Can you work these out from the model? Positions are in its coordinate system, mm. A direction names the side the tool comes from. Give positions to 0.01 mm unless a question says otherwise; leave off trailing zeros. Order: outer loops, then holes, each group sorted by start corner. A loop starts at its lowest first (then second) coordinate and runs counter-clockwise, first axis right, second up.
Item 1: I want a section at C-C, the plane x = -10. Write out the boundary of the cut face in (y, z), then the cut area to 3 significant figures.
Item 2: I want a section at A-A, the plane y = 4.21. Write out the boundary of the cut face in (x, z), then the cut area to 3 significant figures.
Item 3: I want a section at B-B, the plane y = -5. Write out the boundary of the cut face in (x, z), then the cut area to 3 significant figures.
Item 4: If we mould it in two halves opening along X, with no side actions, what happens to faces 3 (the cylindrical face through (5.66, -6.72, 4.06)), 4 (the flat face through (-15, 0, 4)), 5 (the flat face through (0, 7, 4)), 6 (the flat face through (15, 0, 4))? For each: +X half, -X half, draft (parallel to the pull), parting line (faces both ways), or undercut.
Item 5: If I drill on line 1 along X through (y, z) = (4.21, 3.25); line 2 along X through (y, z) = (3.25, 7); line 3 along Y through (x, z) = (-10, 6.25), over which ranges is the centre line in solid material (lowest first)?
Item 6: I want a section at D-D, the plane x = 9.5. Write out the boundary of the cut face in (y, z), then the cut area to 3 significant figures.
Item 7: I'm going to push a flat-ended pin straight in: pin 1 Ø1 at (x, y) = (8.5, 2.5) entering from -Z. Where does the tip first touch, or does it pass through?
Item 8: Which directions (+Z, -Z, +X, -X, +Y, -Y) give clear straight access to the entire face, cutting with the end or side of a thin tool? Please do faces 1 (the flat face through (-14, -7, 4)), 2 (the cylindrical face through (1.01, -6.71, 4.06)).
```python
from build123d import *

# Parameters (mm, degrees)
SKETCH006_W            = 30
SKETCH006_H            = 14
PAD003_DEPTH           = 8
SKETCH007_R            = 3.1
POCKET003_DEPTH        = 0.001
POCKET003_DEPTH_BACK   = 8.001
LINEARPATTERN003_COUNT = 4
LINEARPATTERN003_PITCH = 6.666667
PARTDESIGN_FILLET003_R = 0.5


with BuildPart() as part:
    # Sketch006 → Pad003 (new body)
    with BuildSketch(Plane.XY):
        Rectangle(SKETCH006_W, SKETCH006_H)
    extrude(amount=PAD003_DEPTH)

    # Sketch007 → Pocket003 (cut, two sides)
    with BuildSketch(Plane.XY) as pocket003_sk:
        with Locations((-10, 4.21)):
            Circle(SKETCH007_R)
        with Locations((-10, -4.21)):
            Circle(SKETCH007_R)
    pocket003 = extrude(amount=-POCKET003_DEPTH, mode=Mode.SUBTRACT) + extrude(pocket003_sk.sketch, amount=POCKET003_DEPTH_BACK, mode=Mode.SUBTRACT)

    # LinearPattern003: Pocket003 ×4
    with Locations(*[(i * LINEARPATTERN003_PITCH, 0, 0) for i in range(1, LINEARPATTERN003_COUNT)]):
        add(pocket003, mode=Mode.SUBTRACT)

    # PartDesign__Fillet003
    partdesign_fillet003_edges = [part.edges().sort_by_distance(p)[0] for p in [
        (-15, -7, 4),
        (-15, 7, 4),
        (-11.351259, -7, 4),
        (-11.351259, 7, 4),
        (-6.9, -4.21, 4),
        (-6.9, 4.21, 4),
        (-8.648741, 7, 4),
        (-4.684592, 7, 4),
        (-0.233333, 4.21, 4),
        (-1.982075, 7, 4),
        (1.982075, 7, 4),
        (6.433333, 4.21, 4),
        (4.684592, 7, 4),
        (8.648741, 7, 4),
        (13.1, 4.21, 4),
        (11.351259, 7, 4),
        (15, 7, 4),
        (15, -7, 4),
        (11.351259, -7, 4),
        (13.1, -4.21, 4),
        (8.648741, -7, 4),
        (4.684592, -7, 4),
        (6.433333, -4.21, 4),
        (1.982075, -7, 4),
        (-1.982075, -7, 4),
        (-0.233333, -4.21, 4),
        (-4.684592, -7, 4),
        (-8.648741, -7, 4),
    ]]
    fillet(partdesign_fillet003_edges, radius=PARTDESIGN_FILLET003_R)


solid = part.part
```
Results list:
1. outline: (-1.11, 0) - (1.11, 0) - (1.11, 8) - (-1.11, 8) - close
1. area: 17.8 mm2
2. outline: (-15, 0) - (-13.1, 0) - (-13.1, 8) - (-15, 8) - close; (-6.9, 0) - (-6.43, 0) - (-6.43, 8) - (-6.9, 8) - close; (-0.23, 0) - (0.23, 0) - (0.23, 8) - (-0.23, 8) - close; (6.43, 0) - (6.9, 0) - (6.9, 8) - (6.43, 8) - close; (13.1, 0) - (15, 0) - (15, 8) - (13.1, 8) - close
2. area: 41.6 mm2
3. outline: (-15, 0) - (-13, 0) - (-13, 8) - (-15, 8) - close; (-7, 0) - (-6.33, 0) - (-6.33, 8) - (-7, 8) - close; (-0.34, 0) - (0.34, 0) - (0.34, 8) - (-0.34, 8) - close; (6.33, 0) - (7, 0) - (7, 8) - (6.33, 8) - close; (13, 0) - (15, 0) - (15, 8) - (13, 8) - close
3. area: 48.2 mm2
4. face 3: undercut
4. face 4: -X half
4. face 5: draft
4. face 6: +X half
5. line 1: x = -15 to -13.1, -6.9 to -6.43, -0.23 to 0.23, 6.43 to 6.9, 13.1 to 15
5. line 2: x = -15 to -12.95, -7.05 to -6.28, -0.39 to 0.39, 6.28 to 7.05, 12.95 to 15
5. line 3: y = -1.11 to 1.11
6. outline: (-1.15, 0) - (1.15, 0) - (1.15, 8) - (-1.15, 8) - close
6. area: 18.4 mm2
7. pin 1: passes through
8. face 1: +Z, -Z, +X, -X, -Y
8. face 2: +Z, -Z
